Source: three-view drawing plus pictorial views. Frame: mm from the lowest corner of the part. Give positions to 0.01 mm unless a question says otherwise; leave off trailing zeros. Loops run counter-clockwise (first coordinate to the right, second up) from the corner with the lowest first, then second, coordinate; pieces in that order, holes last. Notation, with made-up numbers: (-21.75, -12.75) - (-0.75, -12.75) arc R6 cw to (-0.75, -1.75) - close; hole circle Ø9 at (70.25, 74). An arc over 180 degrees is marked (long way). One line per item, written item: value.
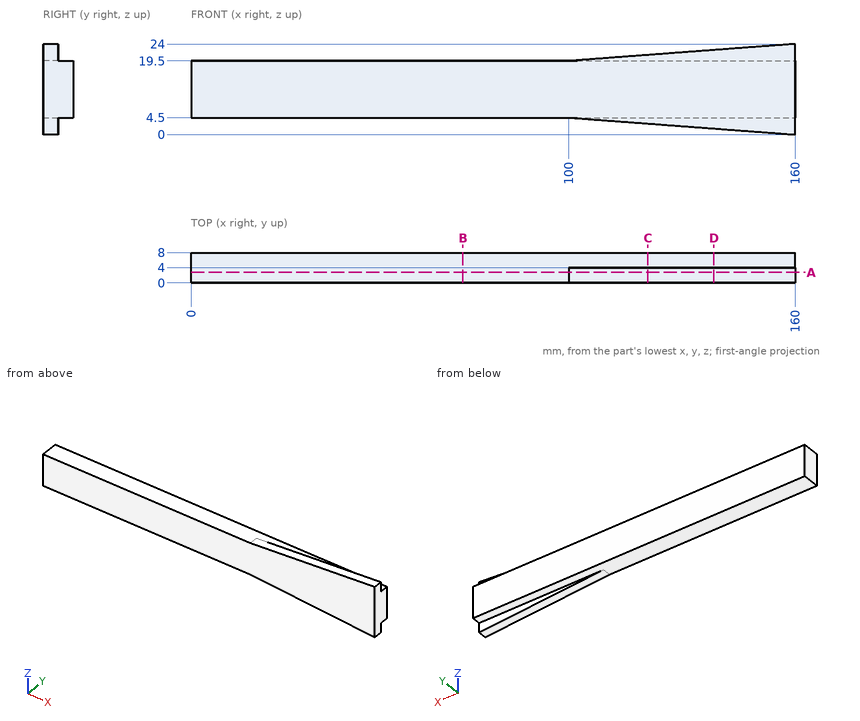
Item 1: Section A-A, the plane y = 2.75. Output: boundary loops of the cut face in (x, z).
Verdict:
outline: (0, 4.5) - (100, 4.5) - (160, 0) - (160, 24) - (100, 19.5) - (0, 19.5) - close
Item 2: Section C-C, the plane x = 121. Output: boundary loops of the cut face in (y, z) (3 decimals).
Verdict:
outline: (0, 2.925) - (4, 2.925) - (4, 4.5) - (8, 4.5) - (8, 19.5) - (4, 19.5) - (4, 21.075) - (0, 21.075) - close
Item 3: Section B-B, the plane x = 72. Output: boundary loops of the cut face in (y, z), and give its area (3 significant figures).
Verdict:
outline: (0, 4.5) - (8, 4.5) - (8, 19.5) - (0, 19.5) - close
area: 120 mm^2
Item 4: Material intervals for L1, parallel to Z at x = 93.5, y = 3.5; L2, parallel to Y at x = 113.5, z = 4; L3, parallel to Z at x = 109, y = 3.5 (3 decimals), sorted ascending.
Verdict:
L1: z = 4.5 to 19.5
L2: y = 0 to 4
L3: z = 3.825 to 20.175
Item 5: Section D-D, the plane x = 138.5. Output: boundary loops of the cut face in (y, z), and give its area (3 significant figures).
Verdict:
outline: (0, 1.61) - (4, 1.61) - (4, 4.5) - (8, 4.5) - (8, 19.5) - (4, 19.5) - (4, 22.39) - (0, 22.39) - close
area: 143 mm^2
Item 6: Pin query (flat end, axial travel): P1, Ø1.4, axis at x = 140.5, z = 2, coming from the +Y side; P2, Ø4, axis at x = 136.5, z = 3, coming from the -Y side; P3, Ø2.5, axis at x = 58.5, y = 2.5, coming from the +Z side. Return the tip coordinate at first contact, or that it passes through.
Verdict:
P1: stops at y = 4
P2: stops at y = 0
P3: stops at z = 19.5
